Build history of the part. All positions in model axes, mm. A direction names the side the tool comes from. Give positions to 0.01 mm unless a question says otherwise; leave off trailing zeros. Write each loop counter-clockwise with the first axis right and the second up, starting at its lowest first coordinate (ties: lowest second). Pieces come first, ordered by that corner, then holes. Notation, with made-up numbers: M -9.75,51 L 49.25,51 A12 cw 49.25,66 Z; hole C 36,-37 d6. An arc over 180 degrees is marked long. Return JSON: item names as keys, results as strings. Group by question number.
Q1. Flat gauge pin, fed straight in: pin 1 Ø12 at (x, z) = (241.3, 0) entering from +Y (3 decimals). Where does the tip first touch, or does it go through?
Q2. Band-saw the part on A-A, the plane x = 139.7. Give the cut face in (y, z) (1 decimal), then the cut area to 3 significant figures.
Q3. Band-saw the part on B-B, the plane x = 232. Give the cut face in (y, z) (3 decimals), then the cut area to 3 significant figures.
Q4. Band-saw the part on C-C, the plane z = 1.5. Count the separate pieces of the cut face and the enclosed holes in it, then the cut area to 3 significant figures.
Q5. Pull direction Z, two halves, no side cores. Call faces 1 (the cylindrical face through (170.334, 0.23, -11.135)), 2 (the cylindrical face through (118.078, -11.135, 0.496)), 3 (the flat face through (125, 0, 12.7)): +Z half, -Z half, draft (parallel to the pull), parting line (faces both ways), or undercut.
Q6. Wall check: probe 1 along Z at (x, y) = (187, 5) (3 decimals); probe 2 along Y at (x, z) = (114.3, 11.45). Give the ranges that are in metal, low to high.
Q7. Tool access for faces 4 (the cylindrical face through (221.88, 11.13, -0.79)), 5 (the cylindrical face through (58.5, 1.57, -11.13)), 6 (the cylindrical face through (34.38, -11.13, 0.83)): list every direction of +Z, -Z, +X, -X, +Y, -Y with a clear straight run to the whole face (end or side of a thin tool).
from build123d import *

# Parameters (mm, degrees)
SKETCH2_W           = 25.4
SKETCH2_H           = 25.4
SKETCH2_W_2         = 19.05
SKETCH2_H_2         = 19.05
BOSS_EXTRUDE1_DEPTH = 254
SKETCH3_R           = 6.0325
CUT_EXTRUDE1_DEPTH  = 3.175
SKETCH4_R           = 3.81
CUT_EXTRUDE2_DEPTH  = 3.175
LPATTERN1_COUNT     = 10
LPATTERN1_PITCH     = 25.4
SKETCH6_R           = 2.2225
CUT_EXTRUDE3_DEPTH  = 3.175
SKETCH7_R           = 5.23875
CUT_EXTRUDE4_DEPTH  = 3.175
LPATTERN2_COUNT     = 10
LPATTERN2_PITCH     = 25.4


with BuildPart() as part:
    # Sketch2 → Boss-Extrude1 (new body)
    with BuildSketch(Plane(origin=(0, 0, 0), x_dir=(0, 0, -1), z_dir=(1, 0, 0))):
        Rectangle(SKETCH2_W, SKETCH2_H)
        Rectangle(SKETCH2_W_2, SKETCH2_H_2, mode=Mode.SUBTRACT)
    extrude(amount=BOSS_EXTRUDE1_DEPTH)

    # Sketch3 → Cut-Extrude1 (cut)
    with BuildSketch(Plane(origin=(0, 12.7, 0), x_dir=(1, 0, 0), z_dir=(0, 1, 0))):
        with Locations(Location((12.7, 0, 0), (0, 0, 270))):
            Circle(SKETCH3_R)
    cut_extrude1 = extrude(amount=-CUT_EXTRUDE1_DEPTH, mode=Mode.SUBTRACT)

    # Sketch4 → Cut-Extrude2 (cut)
    with BuildSketch(Plane.XZ.offset(12.7)):
        with Locations(Location((12.7, 0, 0), (0, 0, 270))):
            Circle(SKETCH4_R)
    cut_extrude2 = extrude(amount=-CUT_EXTRUDE2_DEPTH, mode=Mode.SUBTRACT)

    # LPattern1: Cut-Extrude1, Cut-Extrude2 ×10
    with Locations(*[(i * LPATTERN1_PITCH, 0, 0) for i in range(1, LPATTERN1_COUNT)]):
        add(cut_extrude1, mode=Mode.SUBTRACT)
        add(cut_extrude2, mode=Mode.SUBTRACT)

    # Sketch6 → Cut-Extrude3 (cut)
    with BuildSketch(Plane.XY.offset(12.7)):
        with Locations((12.7, 0)):
            Circle(SKETCH6_R)
    cut_extrude3 = extrude(amount=-CUT_EXTRUDE3_DEPTH, mode=Mode.SUBTRACT)

    # Sketch7 → Cut-Extrude4 (cut)
    with BuildSketch(Plane(origin=(0, 0, -12.7), x_dir=(-1, 0, 0), z_dir=(0, 0, -1))):
        with Locations((-12.7, 0)):
            Circle(SKETCH7_R)
    cut_extrude4 = extrude(amount=-CUT_EXTRUDE4_DEPTH, mode=Mode.SUBTRACT)

    # LPattern2: Cut-Extrude3, Cut-Extrude4 ×10
    with Locations(*[(i * LPATTERN2_PITCH, 0, 0) for i in range(1, LPATTERN2_COUNT)]):
        add(cut_extrude3, mode=Mode.SUBTRACT)
        add(cut_extrude4, mode=Mode.SUBTRACT)


solid = part.part
From the geometry:
{
 "1": {"pin 1": "stops at y = -9.525"},
 "2": {"outline": "M -12.7,-12.7 L -5.2,-12.7 L -5.2,-9.5 L -9.5,-9.5 L -9.5,-3.8 L -12.7,-3.8 Z; M -12.7,3.8 L -9.5,3.8 L -9.5,9.5 L -2.2,9.5 L -2.2,12.7 L -12.7,12.7 Z; M 2.2,9.5 L 9.5,9.5 L 9.5,6 L 12.7,6 L 12.7,12.7 L 2.2,12.7 Z; M 5.2,-12.7 L 12.7,-12.7 L 12.7,-6 L 9.5,-6 L 9.5,-9.5 L 5.2,-9.5 Z", "area": "172 mm^2"},
 "3": {"outline": "M -12.7,-12.7 L 12.7,-12.7 L 12.7,12.7 L -12.7,12.7 Z; hole M -9.525,-9.525 L 9.525,-9.525 L 9.525,9.525 L -9.525,9.525 Z", "area": "282 mm^2"},
 "4": {"separate pieces": "22", "enclosed holes": "0", "area": "1,020 mm^2"},
 "5": {"face 1": "draft", "face 2": "undercut", "face 3": "+Z half"},
 "6": {"probe 1": "z = -12.7 to -9.525, 9.525 to 12.7", "probe 2": "y = -12.7 to -2.22, 2.22 to 12.7"},
 "7": {"face 4": "+Y", "face 5": "-Z", "face 6": "+Y, -Y"}
}
